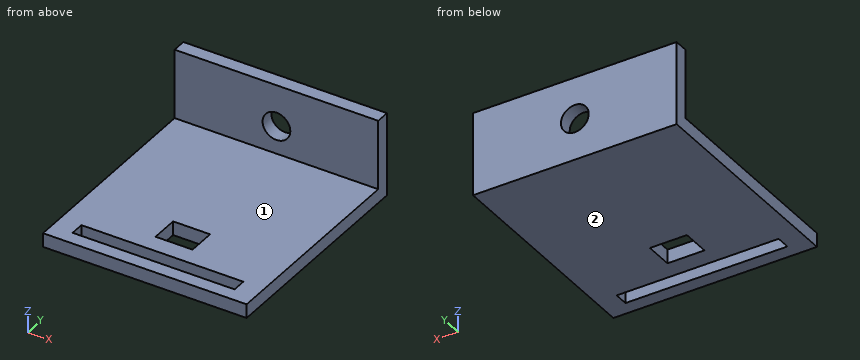
```python
from build123d import *

# Parameters (mm, degrees)
ESTRUSIONE_ESTRUSIONE6_DEPTH = 44
SCHIZZO9_W                   = 35
SCHIZZO9_H                   = 3
TAGLIO_ESTRUSIONE2_DEPTH     = 44
SCHIZZO10_R                  = 3
TAGLIO_ESTRUSIONE3_DEPTH     = 10
SCHIZZO11_W                  = 8
SCHIZZO11_H                  = 6
TAGLIO_ESTRUSIONE4_DEPTH     = 10


with BuildPart() as part:
    # Schizzo8 → Estrusione-Estrusione6 (new body)
    with BuildSketch(Plane(origin=(0, 0, 0), x_dir=(0, 0, -1), z_dir=(1, 0, 0))):
        Polygon((0, 0), (0, 3), (18, 3), (18, -45), (15, -45), (15, 0), align=None)
    extrude(amount=ESTRUSIONE_ESTRUSIONE6_DEPTH)

    # Schizzo9 → Taglio-Estrusione2 (cut)
    with BuildSketch(Plane.XY.offset(-15)):
        with Locations((22, -40.5)):
            Rectangle(SCHIZZO9_W, SCHIZZO9_H)
    extrude(amount=-TAGLIO_ESTRUSIONE2_DEPTH, mode=Mode.SUBTRACT)

    # Schizzo10 → Taglio-Estrusione3 (cut)
    with BuildSketch(Plane(origin=(0, 3, 0), x_dir=(1, 0, 0), z_dir=(0, 1, 0))):
        with Locations((22, 9)):
            Circle(SCHIZZO10_R)
    extrude(amount=-TAGLIO_ESTRUSIONE3_DEPTH, mode=Mode.SUBTRACT)

    # Schizzo11 → Taglio-Estrusione4 (cut)
    with BuildSketch(Plane(origin=(0, 0, -18), x_dir=(-1, 0, 0), z_dir=(0, 0, -1))):
        with Locations((-22, -32)):
            Rectangle(SCHIZZO11_W, SCHIZZO11_H)
    extrude(amount=-TAGLIO_ESTRUSIONE4_DEPTH, mode=Mode.SUBTRACT)


solid = part.part
```
Can you work these out from the model? Positions are in its coordinate system, mm. Face numbers are marked on the shaded views. A direction names the side the tool comes from. Give positions to 0.01 mm unless a question says otherwise; leave off trailing zeros. Order: outer loops, then holes, each group sorted by start corner. A loop starts at its lowest first (then second) coordinate and runs counter-clockwise, first axis right, second up. Notation, with made-up numbers: (-1.75, 20.5) - (7.25, 20.5) arc R19 cw to (7.25, 57.5) - close; hole circle Ø6 at (15.5, 60.25). An arc over 180 degrees is marked (long way). Use a Markdown table: item, result. Add a question column.
Q1. If we section it at D-D on z = -16: Write out the boundary of the cut face in (x, y).
Q2. I'm going to push flat-ended pins straight in: pin 1 (5.5 mm diameter, centred on x = 22, z = -9, fed in from -Y); pin 2 (3 mm diameter, centred on x = 17, y = -31.5, fed in from +Z); pin 3 (5 mm diameter, centred on x = 19, z = -11, fed in from -Y). Where does each tip first touch, or does it pass through?
Q3. On a 3-axis mill with a long thin cutter (end or side, diameter ignored), from which of +Z, -Z, +X, -X, +Y, -Y can I reach the whole of each face in a straight line? I mean the marked faces 1 and 2. Say none if no direction works.
Q4. If we section it at A-A on x = 22: Write out the boundary of the cut face in (y, z).
Q5. Please list where these lines run through material, in increasing order: line 1 along Z through (x, y) = (22, 1.55); line 2 along Z through (x, y) = (12, -36); line 3 along Y through (x, z) = (36, -8.75).
Q6. If we section it at C-C on x = 6: Write out the boundary of the cut face in (y, z).
Q7. If we section it at B-B on z = -9: Write out the boundary of the cut face in (x, y), plus the area to 3 significant figures.
Answers follow:
| question | item | result |
|---|---|---|
| 1 | outline | (0, -45) - (44, -45) - (44, 3) - (0, 3) - close; hole (4.5, -42) - (39.5, -42) - (39.5, -39) - (4.5, -39) - close; hole (18, -35) - (26, -35) - (26, -29) - (18, -29) - close |
| 2 | pin 1 | passes through |
| 2 | pin 2 | stops at z = -15 |
| 2 | pin 3 | stops at y = 0 |
| 3 | face 1 | +Z, +X, -X, -Y |
| 3 | face 2 | -Z, +X, -X, +Y, -Y |
| 4 | outline | (-45, -18) - (-42, -18) - (-42, -15) - (-45, -15) - close; (-39, -18) - (-35, -18) - (-35, -15) - (-39, -15) - close; (-29, -18) - (3, -18) - (3, -12) - (0, -12) - (0, -15) - (-29, -15) - close; (0, -6) - (3, -6) - (3, 0) - (0, 0) - close |
| 5 | line 1 | z = -18 to -12, -6 to 0 |
| 5 | line 2 | z = -18 to -15 |
| 5 | line 3 | y = 0 to 3 |
| 6 | outline | (-45, -18) - (-42, -18) - (-42, -15) - (-45, -15) - close; (-39, -18) - (3, -18) - (3, 0) - (0, 0) - (0, -15) - (-39, -15) - close |
| 7 | outline | (0, 0) - (19, 0) - (19, 3) - (0, 3) - close; (25, 0) - (44, 0) - (44, 3) - (25, 3) - close |
| 7 | area | 114 mm^2 |
